```python
from build123d import *

# Parameters (mm, degrees)
SKETCH1_R           = 21.25
SKETCH1_R_2         = 1.5
BOSS_EXTRUDE1_DEPTH = 5
CHAMFER1_SIZE       = 2.5


with BuildPart() as part:
    # Sketch1 → Boss-Extrude1 (new body)
    with BuildSketch(Plane(origin=(0, 0, 0), x_dir=(1, 0, 0), z_dir=(0, 1, 0))):
        with Locations(Location((0, 0, 0), (0, 0, 270))):
            Circle(SKETCH1_R)
        with Locations(Location((0, 15.5, 0), (0, 0, 270))):
            Circle(SKETCH1_R_2, mode=Mode.SUBTRACT)
        with Locations(Location((15.5, 0, 0), (0, 0, 270))):
            Circle(SKETCH1_R_2, mode=Mode.SUBTRACT)
        with Locations(Location((0, -15.5, 0), (0, 0, 270))):
            Circle(SKETCH1_R_2, mode=Mode.SUBTRACT)
        with Locations(Location((-15.5, 0, 0), (0, 0, 270))):
            Circle(SKETCH1_R_2, mode=Mode.SUBTRACT)
        with BuildLine():
            Line((-1.658312395, 2.5), (1.658312395, 2.5))
            ThreePointArc((1.658312395, 2.5), (0, -3), (-1.658312395, 2.5))
        make_face(mode=Mode.SUBTRACT)
    extrude(amount=BOSS_EXTRUDE1_DEPTH)

    # Chamfer1
    chamfer1_edges = [part.edges().sort_by_distance(p)[0] for p in [
        (0, 5, -21.25),
    ]]
    chamfer(chamfer1_edges, length=CHAMFER1_SIZE)


solid = part.part
```
The model under review builds one solid part; all positions refer to its coordinate system, in mm. A direction names the side the tool comes from. Coordinates: 2 decimals unless noted, no trailing zeros. Write each loop counter-clockwise with the first axis right and the second up, starting at its lowest first coordinate (ties: lowest second). Pieces come first, ordered by that corner, then holes. Notation, with made-up numbers: (40, 73.25) - (99, 73.25) arc R25 ccw to (99, 103.25) - close; hole circle Ø1 at (4, 87). An arc over 180 degrees is marked (long way). Answer in a Markdown table with one row per item. Add a question column.
Q1. Draft analysis for pull direction X (two halves, no side actions). For faces 1 (the face through (-4, 5, 0)), 2 (the face through (16.765, 2.465, 0.806)), 3 (the face through (-12.93, 1.232, -16.863)), 4 (the face through (0, 2, 3)), state which applies: +X half, -X half, draft (parallel to the pull), parting line (faces both ways), or undercut.
Q2. To check wall thickness, follow line 1 along X through (y, z) = (3.3, 0); line 2 along X through (y, z) = (2.75, 0); line 3 along X through (y, z) = (2.45, -10). State the ranges of each line that lie inside material, in increasing order. Write a range as from..to.
Q3. Consider section B-B on x = 0. Give the boundary of the cut face in (y, z), then the cut area to 3 significant figures.
Q4. For faces 5 (the face through (-4, 0, 0)), 6 (the face through (0, 2, -2.5)), list the 3-axis set-ups (+Z, -Z, +X, -X, +Y, -Y) from which the entire face can be reached by the end or side of a thin tool; tool diameter is ignored.
Q5. Consider section A-A on y = 3.4. Give the boundary of the cut face in (x, z).
Q6. Consider section C-C on y = 1.2. Give the boundary of the cut face in (x, z).
Q7. Clearance check with flat-ended pins moving along their axes: pin 1 (1.8 mm diameter, centred on x = 0, z = 15.5, fed in from -Y); pin 2 (5 mm diameter, centred on x = 0, z = -15.5, fed in from -Y); pin 3 (3 mm diameter, centred on x = 4.5, y = 1, fed in from +Z); pin 4 (1 mm diameter, centred on x = -8.5, y = 2, fed in from -Z). State where each tip first meets the part, or that it passes through.
Answers below:
| question | item | result |
|---|---|---|
| 1 | face 1 | draft |
| 1 | face 2 | undercut |
| 1 | face 3 | parting line |
| 1 | face 4 | undercut |
| 2 | line 1 | -20.45..-17, -14..-3, 3..14, 17..20.45 |
| 2 | line 2 | -21..-17, -14..-3, 3..14, 17..21 |
| 2 | line 3 | -18.75..18.75 |
| 3 | outline | (0, -21.25) - (2.5, -21.25) - (5, -18.75) - (5, -17) - (0, -17) - close; (0, -14) - (5, -14) - (5, -2.5) - (0, -2.5) - close; (0, 3) - (5, 3) - (5, 14) - (0, 14) - close; (0, 17) - (5, 17) - (5, 18.75) - (2.5, 21.25) - (0, 21.25) - close |
| 3 | area | 149 mm² |
| 4 | face 5 | +Z, -Z, +X, -X, -Y |
| 4 | face 6 | +Y, -Y |
| 5 | outline | circle Ø40.7 at (0, 0); hole circle Ø3 at (-15.5, 0); hole (-1.66, -2.5) - (1.66, -2.5) arc R3 ccw (long way) to start; hole circle Ø3 at (0, -15.5); hole circle Ø3 at (0, 15.5); hole circle Ø3 at (15.5, 0) |
| 6 | outline | circle Ø42.5 at (0, 0); hole circle Ø3 at (-15.5, 0); hole (-1.66, -2.5) - (1.66, -2.5) arc R3 ccw (long way) to start; hole circle Ø3 at (0, -15.5); hole circle Ø3 at (0, 15.5); hole circle Ø3 at (15.5, 0) |
| 7 | pin 1 | through |
| 7 | pin 2 | y = 0 |
| 7 | pin 3 | z = 21.04 |
| 7 | pin 4 | z = -19.69 |
